from build123d import *

# Parameters (mm, degrees)
BOSS_EXTRUDE1_DEPTH = 22.225
SKETCH2_R           = 2.5
SKETCH2_R_2         = 7.5
CUT_EXTRUDE5_DEPTH  = 18
CUT_EXTRUDE7_START  = 12
SKETCH2_8_R         = 15.5
CUT_EXTRUDE7_DEPTH  = 42


with BuildPart() as part:
    # Sketch1 → Boss-Extrude1 (new body, symmetric)
    with BuildSketch(Plane.XY):
        with BuildLine():
            Line((0, 28), (0, -122))
            ThreePointArc((0, -122), (3.91238571, -129.933533403), (12.588190451, -131.659258263))
            Line((12.588190451, -131.659258263), (49.294095226, -121.823940721))
            ThreePointArc((49.294095226, -121.823940721), (52.263200822, -119.606804413), (52.890738004, -115.954753136))
            Line((52.890738004, -115.954753136), (51.18308621, -107.920883092))
            ThreePointArc((51.18308621, -107.920883092), (47.694814113, -102.228540385), (41.401610203, -100))
            Line((41.401610203, -100), (23, -100))
            ThreePointArc((23, -100), (19.464466094, -98.535533906), (18, -95))
            Line((18, -95), (18, 12))
            ThreePointArc((18, 12), (18.585786438, 13.414213562), (20, 14))
            Line((20, 14), (21, 14))
            ThreePointArc((21, 14), (22.414213562, 14.585786438), (23, 16))
            Line((23, 16), (23, 28))
            Line((23, 28), (18, 28))
            Line((18, 28), (0, 28))
        make_face()
        with BuildLine():
            Line((4, -111), (4, -90))
            ThreePointArc((4, -90), (9, -85), (14, -90))
            Line((14, -90), (14, -111))
            ThreePointArc((14, -111), (9, -116), (4, -111))
        make_face(mode=Mode.SUBTRACT)
        with BuildLine():
            Line((4, -69), (4, -39))
            ThreePointArc((4, -39), (9, -34), (14, -39))
            Line((14, -39), (14, -69))
            ThreePointArc((14, -69), (9, -74), (4, -69))
        make_face(mode=Mode.SUBTRACT)
        with BuildLine():
            Line((29.708099244, -108.5), (36.291900756, -108.5))
            ThreePointArc((36.291900756, -108.5), (44, -110), (36.291900756, -111.5))
            Line((36.291900756, -111.5), (29.708099244, -111.5))
            ThreePointArc((29.708099244, -111.5), (22, -110), (29.708099244, -108.5))
        make_face(mode=Mode.SUBTRACT)
        Polygon((4, 12), (4, -12), (12, -14.5), (12, 14.5), align=None, mode=Mode.SUBTRACT)
    extrude(amount=BOSS_EXTRUDE1_DEPTH, both=True)

    # Sketch2 → Cut-Extrude5 (cut)
    with BuildSketch(Plane(origin=(0, 0, 0), x_dir=(0, 0, -1), z_dir=(1, 0, 0))):
        with Locations((14, -78)):
            Circle(SKETCH2_R)
        with Locations((-14, -78)):
            Circle(SKETCH2_R)
        with Locations((-14, -25)):
            Circle(SKETCH2_R)
        with Locations((14, -25)):
            Circle(SKETCH2_R)
        Circle(SKETCH2_R_2)
    extrude(amount=CUT_EXTRUDE5_DEPTH, mode=Mode.SUBTRACT)

    # Sketch2<8> → Cut-Extrude7 (cut, through all)
    with BuildSketch(Plane(origin=(0, 0, 0), x_dir=(0, 0, -1), z_dir=(1, 0, 0)).offset(CUT_EXTRUDE7_START)):
        Circle(SKETCH2_8_R)
    extrude(amount=CUT_EXTRUDE7_DEPTH, mode=Mode.SUBTRACT)


solid = part.part
Here's how the part is built. I have some questions about the finished solid (model axes, mm). A direction names the side the tool comes from. Give positions to 0.01 mm unless a question says otherwise; leave off trailing zeros. Loops run counter-clockwise (first coordinate to the right, second up) from the corner with the lowest first, then second, coordinate; pieces in that order, holes last. Notation, with made-up numbers: (32.5, 88.25) -> (52.5, 88.25) arc R17 ccw to (52.5, 117.25) -> close; hole circle Ø3 at (27.5, 81). An arc over 180 degrees is marked (long way). Answer as a JSON object with one key per item and string values. Group by question number.
Item 1: Will these pins go through, and if not, where does the flat tip stop? pin 1 (3 mm diameter, centred on x = 23, z = 4, fed in from -Y); pin 2 (5.5 mm diameter, centred on x = 34.5, z = -11, fed in from +Y); pin 3 (5.5 mm diameter, centred on x = 34, z = 7.5, fed in from -Y); pin 4 (10.5 mm diameter, centred on x = 26, y = -110, fed in from +Z) (3 decimals).
Item 2: Imagine slicing it at D-D on z = -19. Give the number of separate pieces and of enclosed holes in the cut face, then the cut area to 3 significant figures.
Item 3: On a 3-axis mill with a long thin cutter (end or side, diameter ignored), from which of +Z, -Z, +X, -X, +Y, -Y can I reach the whole of each face in a straight line? I mean faces 3 (the flat face through (33, -111.5, 0)), 4 (the cylindrical face through (14.963, 15.368, 2.018)), 5 (the flat face through (23, 22, 0)), 6 (the cylindrical face through (20, -99, 0)). Say none if no direction works.
Item 4: I need wall thicknesses on L1, parallel to Z at x = 1.6, y = 0 (3 decimals); L2, parallel to X at y = -57.5, z = -4.5; L3, parallel to Y at x = 5, z = -14. Which ranges of each line are inside material? Lowest first, please.
Item 5: Imagine slicing it at C-C on y = 0. Write out the boundary of the cut face in (x, z) (3 decimals).
Item 6: Thinking about a two-plate mould opening in Z: for faces 1 (the cylindrical face through (44, -110, 0)), 2 (the cylindrical face through (8.87, -23.31, -12.16)), which applies, pulls with the +Z half, pulls with the -Z half, needs draft (parallel to the pull), parting line crosses it, or undercut?
Item 7: Imagine slicing it at B-B on x = 9. Write out the boundary of the cut face in (y, z) (1 decimal), then the cut area to 3 significant figures.
Item 8: Imagine slicing it at A-A on y = -25. Write out the boundary of the cut face in (x, z) (3 decimals), then the cut area to 3 significant figures.
Answer list:
{
 "1": {"pin 1": "stops at y = -129.27", "pin 2": "stops at y = -100", "pin 3": "stops at y = -126.66", "pin 4": "stops at z = 22.225"},
 "2": {"separate pieces": "1", "enclosed holes": "4", "area": "2,780 mm2"},
 "3": {"face 3": "+Z, -Z", "face 4": "+X", "face 5": "+Z, -Z, +X, +Y", "face 6": "+Z, -Z, +X"},
 "4": {"L1": "z = -22.225 to -7.5, 7.5 to 22.225", "L2": "x = 0 to 4, 14 to 18", "L3": "y = -130.66 to -114, -87 to -80.5, -75.5 to -72, -36 to -27.5, -22.5 to -12.31, 12.31 to 28"},
 "5": {"outline": "(0, -22.225) -> (4, -22.225) -> (4, -7.5) -> (0, -7.5) -> close; (0, 7.5) -> (4, 7.5) -> (4, 22.225) -> (0, 22.225) -> close; (12, -22.225) -> (18, -22.225) -> (18, -15.5) -> (12, -15.5) -> close; (12, 15.5) -> (18, 15.5) -> (18, 22.225) -> (12, 22.225) -> close"},
 "6": {"face 1": "needs draft", "face 2": "undercut"},
 "7": {"outline": "(-131.9, -22.2) -> (-116, -22.2) -> (-116, 22.2) -> (-131.9, 22.2) -> close; (-85, -22.2) -> (-74, -22.2) -> (-74, 22.2) -> (-85, 22.2) -> close; (-34, -22.2) -> (-13.6, -22.2) -> (-13.6, 22.2) -> (-34, 22.2) -> close; (13.6, -22.2) -> (28, -22.2) -> (28, 22.2) -> (13.6, 22.2) -> close; hole circle Ø5 at (-78, -14); hole circle Ø5 at (-78, 14); hole circle Ø5 at (-25, -14); hole circle Ø5 at (-25, 14)", "area": "2,670 mm2"},
 "8": {"outline": "(0, -22.225) -> (18, -22.225) -> (18, -16.5) -> (0, -16.5) -> close; (0, -11.5) -> (18, -11.5) -> (18, 11.5) -> (0, 11.5) -> close; (0, 16.5) -> (18, 16.5) -> (18, 22.225) -> (0, 22.225) -> close", "area": "620 mm2"}
}
